Autodesk Inventor part; units mm, degrees
ref_plane "YZ Plane" through (0, 0, 0) normal (1, 0, 0) x (0, 1, 0)
ref_plane "XZ Plane" through (0, 0, 0) normal (0, 1, 0) x (-1, 0, 0)
ref_plane "XY Plane" through (0, 0, 0) normal (0, 0, 1) x (1, 0, 0)
sketch "Sketch1" plane through (0, 0, 0) normal (0, 0, 1) x (1, 0, 0)
  circle A0 centre (0, 24.7) radius 8.1
  line L0 (0, 24.7) -> (0, 0) construction
  line L1 (0, 0) -> (-20, 0) construction
  line L2 (-20, 5) -> (-9.2, 5)
  line L3 (-9.2, 5) -> (-3.85, 17.5735)
  line L4 (0, 0) -> (20, 0) construction
  line L5 (20, 0) -> (20, 5) construction
  line L6 (20, 5) -> (9.2, 5)
  line L7 (9.2, 5) -> (3.85, 17.5735)
  line L8 (0, 24.7) -> (0, 32.8) construction
  line L9 (-3.85, 17.5735) -> (3.85, 17.5735) construction
  line L10 (-20, 5) -> (-20, 42)
  line L11 (-20, 42) -> (20, 42)
  line L12 (20, 42) -> (20, 5)
  line L13 (-20, 5) -> (-20, 0)
  line L14 (-20, 0) -> (20, 0)
  line L15 (20, 0) -> (20, 5)
  line L16 (-9.2, 5) -> (9.2, 5)
  point P0 (0, 42)
  point P1 (-20, 5)
  dimension "d0" = 16.2
  dimension "d2" = 5
  dimension "d5" = 7.7
  dimension "d91" = 42
  dimension "d102" = 19.7
  dimension "d103" = 18.4
  dimension "d104" = 40
extrude "Extrusion1" add sketch "Sketch1" along normal blind 30 contours A0 L3 L2 L10 L11 L12 L6 L7
extrude "Extrusion2" add sketch "Sketch1" against normal blind 10
sketch "Sketch6" plane through (-20, 42, 30) normal (0, 1, 0) x (1, 0, 0)
  line L0 (0, 40) -> (0, 0)
  line L1 (40, 0) -> (0, 0)
  line L2 (0, 40) -> (40, 0) construction
  line L3 (40, 40) -> (0, 0) construction
  circle A0 centre (35, 5) radius 1.5
  circle A1 centre (5, 5) radius 1.5
  circle A2 centre (5, 35) radius 1.5
  circle A3 centre (35, 35) radius 1.5
  line L4 (35, 35) -> (35, 5) construction
  line L5 (5, 5) -> (35, 5) construction
  line L6 (5, 5) -> (5, 35) construction
  circle A4 centre (20, 20) radius 1.5
  line L7 (40, 40) -> (40, 0)
  line L8 (0, 40) -> (40, 40)
  point P0 (20, 30)
  dimension "d69" = 30
  dimension "d70" = 3
  dimension "d73" = 3
extrude "Extrusion8" cut sketch "Sketch6" against normal blind 5 contours A0 | A1 | A2 | A3
extrude "Extrusion9" cut sketch "Sketch6" against normal through all contours A4
sketch "Sketch8" plane through (20, 5, 30) normal (1, 0, 0) x (0, 0, -1)
  line L0 (0, 0) -> (0, 37)
  line L1 (30, 0) -> (0, 0)
  line L2 (20, 37) -> (20, 15) construction
  line L3 (20, 15) -> (10, 15) construction
  line L4 (20, 15) -> (30, 15) construction
  circle A0 centre (10, 15) radius 1.75
  circle A1 centre (30, 15) radius 1.75
  line L5 (40, 37) -> (0, 37)
  line L6 (30, -5) -> (30, 0)
  line L7 (30, -5) -> (40, -5)
  line L8 (40, 37) -> (40, -5)
  point P0 (30, -5)
  point P1 (35, -5)
  dimension "d97" = 3.5
  dimension "d98" = 3.5
  dimension "d105" = 20
  dimension "d106" = 20
  dimension "d107" = 20
extrude "Extrusion12" cut sketch "Sketch8" against normal blind 5 contours A0 | A1
mirror "Mirror1" about plane through (0, 0, 0) normal (1, 0, 0) of "Extrusion12"
properties part number "X Axis End_3DPrint"
The model under review builds one solid part; all positions refer to its coordinate system, in mm. A direction names the side the tool comes from. Coordinates: 2 decimals unless noted, no trailing zeros. Write each loop counter-clockwise with the first axis right and the second up, starting at its lowest first coordinate (ties: lowest second). Pieces come first, ordered by that corner, then holes. Notation, with made-up numbers: (11.25, 78) - (57.25, 78) arc R19 ccw to (57.25, 100) - close; hole circle Ø7 at (56, -14). An arc over 180 degrees is marked (long way). Write item = value, one per line.
(1) Consider section C-C, the plane z = 10. Give the boundary of the cut face in (x, y), then the cut area to 3 significant figures.
Result sheet:
outline = (-20, 5) - (-9.2, 5) - (-3.85, 17.57) arc R8.1 cw to (-1.5, 32.66) - (-1.5, 42) - (-20, 42) - close; (1.5, 32.66) arc R8.1 cw to (3.85, 17.57) - (9.2, 5) - (20, 5) - (20, 42) - (1.5, 42) - close
area = 1,090 mm^2
(2) Machinability: for faces 1 (the face through (-16.11, 39.53, 23.99)), 2 (the face through (-15, 5, 15)), 3 (the face through (-15, 20, 20)), 4 (the face through (17.54, 21.18, 21.29)), 5 (the face through (-0.3, 32.794, 14.79)), which of the approach directions +Z, -Z, +X, -X, +Y, -Y give a long, thin tool a straight path to every point of the face, cutting with its end or side? Answer none if there is none.
Result sheet:
face_1 = +Y
face_2 = +Z, +X, -X, -Y
face_3 = -X
face_4 = +X
face_5 = +Z
(3) Mouldability with a two-part tool opening along Z and no side actions: class faces 6 (the face through (0, 21, -10)), 7 (the face through (0, 13, 0)), 8 (the face through (13.5, 39.53, -5.07)), 9 (the face through (-6.56, 11.2, 14.79)) as pulls with the +Z half, pulls with the -Z half, needs draft (parallel to the pull), parting line crosses it, or undercut.
Result sheet:
face_6 = pulls with the -Z half
face_7 = pulls with the +Z half
face_8 = undercut
face_9 = needs draft
(4) For P1, Ø3.5, axis at x = 0, z = 10, coming from the -Y side; P2, Ø6, axis at x = 0, y = 18, coming from the +Z side; P3, Ø1, axis at y = 19.5, z = -0.5, coming from the +X side, all flat-tipped, find the tip position at first contact; note any pin that passes through.
Result sheet:
P1 = 32.61
P2 = 0
P3 = 15
(5) Consider section A-A, the plane x = 0. Give the boundary of the cut face in (y, z).
Result sheet:
outline = (0, -10) - (42, -10) - (42, 8.5) - (32.8, 8.5) - (32.8, 0) - (0, 0) - close; (32.8, 11.5) - (42, 11.5) - (42, 30) - (32.8, 30) - close
(6) Consider section D-D, the plane x = -12.5. Give the boundary of the cut face in (y, z), then the cut area to 3 significant figures.
Result sheet:
outline = (0, -10) - (42, -10) - (42, 30) - (5, 30) - (5, 0) - (0, 0) - close
area = 1,530 mm^2
(7) Consider section B-B, the plane y = 38. Give the boundary of the cut face in (x, z).
Result sheet:
outline = (-20, -10) - (20, -10) - (20, 30) - (-20, 30) - close; hole circle Ø3 at (-15, -5); hole circle Ø3 at (-15, 25); hole circle Ø3 at (0, 10); hole circle Ø3 at (15, -5); hole circle Ø3 at (15, 25)
(8) For line 1 (Z direction, x = -15, y = 38); line 2 (X direction, y = 38.55, z = -5); line 3 (X direction, y = 35.25, z = 10), list the stretches that pass through material, from the lowest coordinate up. Write a range as [from, to].
Result sheet:
line_1 = [-10, -6.5], [-3.5, 23.5], [26.5, 30]
line_2 = [-20, -16.5], [-13.5, 13.5], [16.5, 20]
line_3 = [-20, -1.5], [1.5, 20]
